Autodesk Inventor part; units mm, degrees
ref_plane "YZ Plane" through (0, 0, 0) normal (1, 0, 0) x (0, 1, 0)
ref_plane "XZ Plane" through (0, 0, 0) normal (0, 1, 0) x (-1, 0, 0)
ref_plane "XY Plane" through (0, 0, 0) normal (0, 0, 1) x (1, 0, 0)
sketch "Boceto1" plane through (0, 0, 0) normal (0, 1, 0) x (-1, 0, 0)
  circle A0 centre (4.9618, 13.8747) radius 6.35
  dimension "d0" = 12.7
extrude "Extrusión1" add sketch "Boceto1" along normal blind 434
sketch "Boceto2" plane through (-4.9618, 434, 13.8747) normal (0, 1, 0) x (1, 0, 0)
  circle A0 centre (0, 0) radius 3
  point P0 (4.9618, 13.8747)
  dimension "d3" = 6
hole "Agujero1" at (-4.9618, 434, 13.8747) direction (0, -1, 0) diameter 6 depth 15 tip angle 118
sketch "Boceto3" plane through (-4.9618, 0, 13.8747) normal (0, -1, 0) x (1, 0, 0)
  circle A0 centre (0, 0) radius 3
  point P0 (4.9618, -13.8747)
  dimension "d11" = 6
hole "Agujero2" at (-4.9618, 0, 13.8747) direction (0, 1, 0) diameter 6 depth 15 tip angle 118
thread "Thread1"
thread "Thread2"
sketch "Boceto4" plane through (-4.9618, 434, 13.8747) normal (0, 1, 0) x (1, 0, 0)
  circle A0 centre (0, 0) radius 4
  circle A1 centre (0, 0) radius 7
  dimension "d23" = 8
  dimension "d30" = 14
sketch "Boceto5" plane through (-4.9618, 0, 13.8747) normal (0, -1, 0) x (1, 0, 0)
  circle A0 centre (0, 0) radius 4
  circle A1 centre (0, 0) radius 6.5
  dimension "d24" = 8
  dimension "d29" = 13
extrude "Extrusión2" cut sketch "Boceto5" against normal blind 10
extrude "Extrusión3" cut sketch "Boceto4" against normal blind 10
properties part number "Guias de mesa" material "Steel, High Strength, Low Alloy"
Can you work these out from the model? Positions are in its coordinate system, mm. A direction names the side the tool comes from. Give positions to 0.01 mm unless a question says otherwise; leave off trailing zeros. Loops run counter-clockwise (first coordinate to the right, second up) from the corner with the lowest first, then second, coordinate; pieces in that order, holes last. Notation, with made-up numbers: (11.5, 72.5) - (57.5, 72.5) arc R20 cw to (57.5, 89.5) - close; hole circle Ø4 at (11, 45). An arc over 180 degrees is marked (long way). One line per item, written item: value.
(1) On a 3-axis mill with a long thin cutter (end or side, diameter ignored), from which of +Z, -Z, +X, -X, +Y, -Y can I reach the whole of each face in a straight line? I mean faces 1 (the face through (-0.8, 10, 14)), 2 (the face through (-0.8, 424, 13.8)), 3 (the face through (-6, 434, 17)). Say none if no direction works.
Verdict:
face 1: -Y
face 2: +Y
face 3: +Z, -Z, +X, -X, +Y
(2) I need wall thicknesses on line 1 along Z through (x, y) = (-6, 84.5); line 2 along Y through (x, z) = (-0.75, 16); line 3 along Z through (x, y) = (0, 293.5). Which ranges of each line are inside material? Lowest first, please.
Verdict:
line 1: 7.61 to 20.14
line 2: 10 to 424
line 3: 9.91 to 17.84
(3) I'm going to push flat-ended pins straight in: pin 1 (5 mm diameter, centred on x = -9, y = 248, fed in from -Z); pin 2 (2 mm diameter, centred on y = 225, z = 9, fed in from +X); pin 3 (3.5 mm diameter, centred on x = -4.96, z = 13.87, fed in from +Y). Where does each tip first touch, or does it pass through?
Verdict:
pin 1: z = 7.71
pin 2: x = 0.07
pin 3: y = 418.25
(4) If we section it at A-A, the plane y = 341.5: List the corners of the cut face in (x, z) for me.
Verdict:
outline: circle Ø12.7 at (-4.96, 13.87)
